Part model, mm, in its own coordinate system. A direction names the side the tool comes from. Coordinates: 2 decimals unless noted, no trailing zeros. Loops run counter-clockwise (first coordinate to the right, second up) from the corner with the lowest first, then second, coordinate; pieces in that order, holes last.
```python
from build123d import *

# Parameters (mm, degrees)
SKETCH1_W           = 85.6
SKETCH1_H           = 52.98
BOSS_EXTRUDE1_DEPTH = 2.6
SKETCH2_R           = 13.375
CUT_EXTRUDE1_DEPTH  = 2.2
SKETCH3_R           = 12
CUT_EXTRUDE2_DEPTH  = 1.75
FILLET1_R           = 5
CUT_EXTRUDE3_START  = -0.5
CUT_EXTRUDE3_DEPTH  = 0.5


# Read off the part's stored shape, not the designer's step: Cut-Extrude3
with BuildPart() as part:
    # Sketch1 → Boss-Extrude1 (new body)
    with BuildSketch(Plane(origin=(0, 0, 0), x_dir=(1, 0, 0), z_dir=(0, 1, 0))):
        Rectangle(SKETCH1_W, SKETCH1_H)
    extrude(amount=BOSS_EXTRUDE1_DEPTH)

    # Sketch2 → Cut-Extrude1 (cut)
    with BuildSketch(Plane(origin=(0, 2.6, 0), x_dir=(1, 0, 0), z_dir=(0, 1, 0))):
        with Locations(Location((-25.8, 9.49, 0), (0, 0, 270))):
            Circle(SKETCH2_R)
        with Locations(Location((0, -9.51, 0), (0, 0, 270))):
            Circle(SKETCH2_R)
        with Locations(Location((25.8, 9.49, 0), (0, 0, 270))):
            Circle(SKETCH2_R)
    extrude(amount=-CUT_EXTRUDE1_DEPTH, mode=Mode.SUBTRACT)

    # Sketch3 → Cut-Extrude2 (cut)
    with BuildSketch(Plane(origin=(0, 0.4, 0), x_dir=(1, 0, 0), z_dir=(0, 1, 0))):
        with Locations(Location((-25.8, 9.49, 0), (0, 0, 270))):
            Circle(SKETCH3_R)
        with Locations(Location((0, -9.51, 0), (0, 0, 270))):
            Circle(SKETCH3_R)
        with Locations(Location((25.8, 9.49, 0), (0, 0, 270))):
            Circle(SKETCH3_R)
    extrude(amount=-CUT_EXTRUDE2_DEPTH, mode=Mode.SUBTRACT)

    # Fillet1
    fillet1_edges = [part.edges().sort_by_distance(p)[0] for p in [
        (42.8, 1.3, 26.49),
        (-42.8, 1.3, 26.49),
        (-42.8, 1.3, -26.49),
        (42.8, 1.3, -26.49),
    ]]
    fillet(fillet1_edges, radius=FILLET1_R)

    # Cut-Extrude3 outline → Cut-Extrude3 (cut)
    with BuildSketch(Plane(origin=(0, 2.6, 0), x_dir=(1, 0, 0), z_dir=(0, 1, 0)).offset(CUT_EXTRUDE3_START)):
        Polygon((-5, 23), (-5, 8), (5, 8), (5, 10), (-3, 10), (-3, 23), align=None)
    extrude(amount=CUT_EXTRUDE3_DEPTH, mode=Mode.SUBTRACT)


solid = part.part
```
Q1. Drop a flat-ended pin along its axis: P1, Ø5, axis at x = 0, z = -3.5, coming from the +Y side. Give the stop position or say it passes through.
Q2. Saw through at D-D (z = 0.5). List the corners of the cut face in (x, y).
Q3. Saw through at C-C (y = 1.6). List the corners of the cut face in (x, z) (3 decimals), plus the area to 3 significant figures.
Q4. Probe line 1 (X direction, y = 0.3, z = -9.49); line 2 (X direction, y = 1.15, z = -9.49) (3 decimals); line 3 (X direction, y = 1.55, z = 9.51) (3 decimals). List the from-to ranges inside material, lowest first.
Q5. Saw through at A-A (z = 9.5). List the corners of the cut face in (x, y) (3 decimals), plus the area to 3 significant figures.
Q6. Tool access for faces 1 (the cylindrical face through (-37.515, 0.203, -12.091)), 2 (the cylindrical face through (12.743, 1.515, -12.389)): list every direction of +Z, -Z, +X, -X, +Y, -Y with a clear straight run to the whole face (end or side of a thin tool).
Q7. Saw through at B-B (x = 25.8). List the corners of the cut face in (y, z) (3 decimals).
Q8. Mould opens along X. For faces 3 (the flat face through (-42.8, 1, 0)), 4 (the cylindrical face through (37.7, 0.2, -11.05)), 5 (the cylindrical face through (41.3, 1.32, 25.06)), 6 (the flat face through (-1, 0, -6)) say: released by +X, released by -X, zero draft, split by the parting line, or undercut.
Checked values:
1. P1: stops at y = 2.6
2. outline: (-42.8, 0) - (-32.45, 0) - (-32.45, 0.4) - (-34.69, 0.4) - (-34.69, 2.6) - (-42.8, 2.6) - close; (-19.15, 0) - (-7.93, 0) - (-7.93, 0.4) - (-9.88, 0.4) - (-9.88, 2.6) - (-16.91, 2.6) - (-16.91, 0.4) - (-19.15, 0.4) - close; (7.93, 0) - (19.15, 0) - (19.15, 0.4) - (16.91, 0.4) - (16.91, 2.6) - (9.88, 2.6) - (9.88, 0.4) - (7.93, 0.4) - close; (32.45, 0) - (42.8, 0) - (42.8, 2.6) - (34.69, 2.6) - (34.69, 0.4) - (32.45, 0.4) - close
3. outline: (-42.8, -21.49) arc R5 ccw to (-37.8, -26.49) - (37.8, -26.49) arc R5 ccw to (42.8, -21.49) - (42.8, 21.49) arc R5 ccw to (37.8, 26.49) - (-37.8, 26.49) arc R5 ccw to (-42.8, 21.49) - close; hole circle Ø26.75 at (-25.8, -9.49); hole circle Ø26.75 at (0, 9.51); hole circle Ø26.75 at (25.8, -9.49)
3. area: 2,830 mm2
4. line 1: x = -42.8 to -37.8, -13.8 to 13.8, 37.8 to 42.8
4. line 2: x = -42.8 to -39.175, -12.425 to 12.425, 39.175 to 42.8
4. line 3: x = -42.8 to -13.375, 13.375 to 42.8
5. outline: (-42.8, 0) - (-12, 0) - (-12, 0.4) - (-13.375, 0.4) - (-13.375, 2.6) - (-42.8, 2.6) - close; (12, 0) - (42.8, 0) - (42.8, 2.6) - (13.375, 2.6) - (13.375, 0.4) - (12, 0.4) - close
5. area: 154 mm2
6. face 1: +Y, -Y
6. face 2: +Y
7. outline: (0, -26.49) - (2.6, -26.49) - (2.6, -22.865) - (0.4, -22.865) - (0.4, -21.49) - (0, -21.49) - close; (0, 2.51) - (0.4, 2.51) - (0.4, 3.885) - (2.6, 3.885) - (2.6, 26.49) - (0, 26.49) - close
8. face 3: released by -X
8. face 4: undercut
8. face 5: released by +X
8. face 6: zero draft
